```python
from build123d import *

# Parameters (mm, degrees)
CROQUIS_PCB_W    = 88
CROQUIS_PCB_H    = 50
PCB_DEPTH        = 1.6
CROQUIS_ESP32_W  = 28.3
CROQUIS_ESP32_H  = 51.5
ESP32_DEPTH      = 14
CROQUIS_INA219_W = 23
CROQUIS_INA219_H = 20.3
INA219_DEPTH     = 12


with BuildPart() as part:
    # Croquis_pcb → PCB (new body)
    with BuildSketch(Plane(origin=(0, 0, 0), x_dir=(1, 0, 0), z_dir=(0, 1, 0))):
        Rectangle(CROQUIS_PCB_W, CROQUIS_PCB_H)
    extrude(amount=PCB_DEPTH)

    # Croquis_esp32 → ESP32 (add)
    with BuildSketch(Plane(origin=(0, 1.6, 0), x_dir=(1, 0, 0), z_dir=(0, 1, 0))):
        with Locations((9.3, 1.22)):
            Rectangle(CROQUIS_ESP32_W, CROQUIS_ESP32_H)
    extrude(amount=ESP32_DEPTH)

    # Croquis_ina219 → INA219 (add)
    with BuildSketch(Plane(origin=(0, 1.6, 0), x_dir=(1, 0, 0), z_dir=(0, 1, 0))):
        with Locations((-25.1, -12.75)):
            Rectangle(CROQUIS_INA219_W, CROQUIS_INA219_H)
    extrude(amount=INA219_DEPTH)


solid = part.part
```
Here's how the part is built. I have some questions about the finished solid (model axes, mm). A direction names the side the tool comes from. Give positions to 0.01 mm unless a question says otherwise; leave off trailing zeros. Loops run counter-clockwise (first coordinate to the right, second up) from the corner with the lowest first, then second, coordinate; pieces in that order, holes last. Notation, with made-up numbers: M -23.5,-35 L 29.5,-35 A32 ccw 29.5,-1 Z; hole C -17.5,-14 d10. An arc over 180 degrees is marked long. Use one line per item in the form item = value. Start each with the question number.
Q1. If we section it at C-C (x = -10): Write out the boundary of the cut face in (y, z).
Q2. If we section it at A-A (y = 6.25): Write out the boundary of the cut face in (x, z), then the cut area to 3 significant figures.
Q3. Thinking about a two-plate mould opening in X: for faces 4 (the flat face through (-4.85, 9, -1)), 5 (the flat face through (9, 9, -26.97)), 6 (the flat face through (-36.6, 8, 13)), which applies, +X half, -X half, draft (parallel to the pull), parting line (faces both ways), or undercut?
Q4. Which directions (+Z, -Z, +X, -X, +Y, -Y) give clear straight access to the entire face, cutting with the end or side of a thin tool? Please do faces 1 (the flat face through (-25, 13.6, 13)), 2 (the flat face through (23.45, 9, -1)), 3 (the flat face through (9, 9, 24.53)).
Q5. If we section it at B-B (z = 9): Write out the boundary of the cut face in (x, y).
Q6. If we section it at D-D (z = -7.5): Write out the boundary of the cut face in (x, y).
Q7. I need wall thicknesses on line 1 along X through (y, z) = (12.25, 9); line 2 along Y through (x, z) = (-21, -9); line 3 along Y through (x, z) = (-36.5, 5). Which ranges of each line are inside material? Lowest first, please.
Q8. Will these pins go through, and if not, where does the flat tip stop? pin 1 Ø0.5 at (x, y) = (13.5, 1) entering from -Z; pin 2 Ø3.5 at (x, y) = (-27, 8.5) entering from -Z; pin 3 Ø8 at (y, z) = (10, 10) entering from +X; pin 4 Ø6 at (y, z) = (3, 17.5) entering from -X.
Taken from the geometry:
q1.outline = M 0,-25 L 1.6,-25 L 1.6,25 L 0,25 Z
q2.outline = M -36.6,2.6 L -13.6,2.6 L -13.6,22.9 L -36.6,22.9 Z; M -4.85,-26.97 L 23.45,-26.97 L 23.45,24.53 L -4.85,24.53 Z
q2.area = 1,920 mm^2
q3.face_4 = undercut
q3.face_5 = draft
q3.face_6 = -X half
q4.face_1 = +Z, -Z, -X, +Y
q4.face_2 = +Z, -Z, +X, +Y
q4.face_3 = +Z, +X, -X, +Y
q5.outline = M -44,0 L 44,0 L 44,1.6 L 23.45,1.6 L 23.45,15.6 L -4.85,15.6 L -4.85,1.6 L -13.6,1.6 L -13.6,13.6 L -36.6,13.6 L -36.6,1.6 L -44,1.6 Z
q6.outline = M -44,0 L 44,0 L 44,1.6 L 23.45,1.6 L 23.45,15.6 L -4.85,15.6 L -4.85,1.6 L -44,1.6 Z
q7.line_1 = -36.6 to -13.6, -4.85 to 23.45
q7.line_2 = 0 to 1.6
q7.line_3 = 0 to 13.6
q8.pin_1 = -25
q8.pin_2 = 2.6
q8.pin_3 = 23.45
q8.pin_4 = -44
